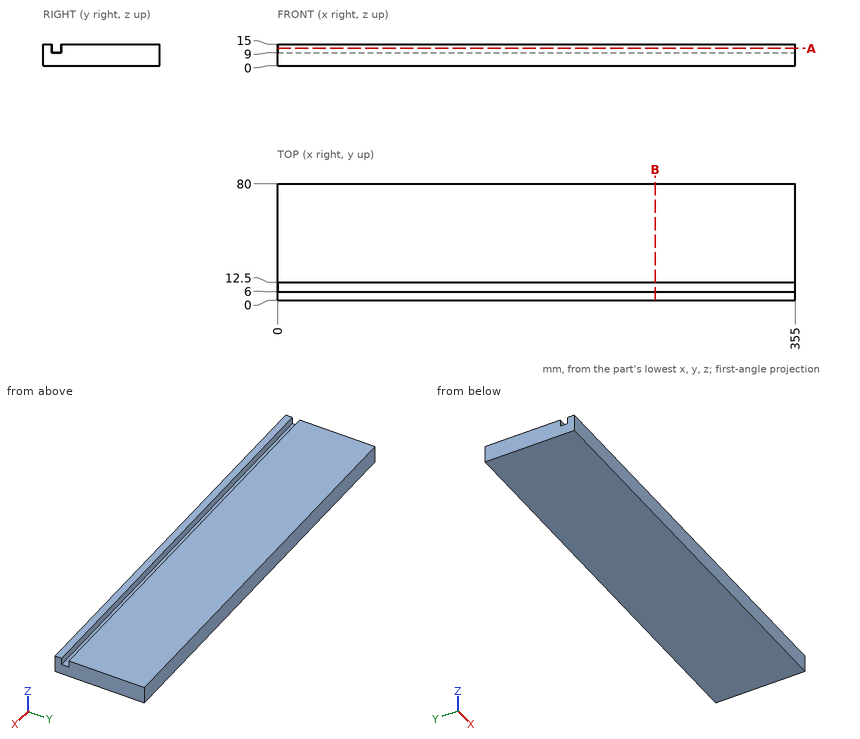
The figure shows three views and two pictorial views of one solid part (mm, origin at its lowest corner). Answer the questions. Round coordinates to 2 decimals unless told otherwise and drop trailing zeros. Loops run counter-clockwise (first coordinate to the right, second up) from the corner with the lowest first, then second, coordinate; pieces in that order, holes last. Notation, with made-up numbers: (15.25, 84.5) -> (53.25, 84.5) arc R19 cw to (53.25, 102.5) -> close; hole circle Ø10 at (-20, 7.5). An arc over 180 degrees is marked (long way). Use one line per item in the form item = value.
(1) Find section A-A on z = 12. Give the vertices of the cut face in (x, y), then the cut area to 3 significant figures.
Answer list:
outline = (0, 0) -> (355, 0) -> (355, 6) -> (0, 6) -> close; (0, 12.5) -> (355, 12.5) -> (355, 80) -> (0, 80) -> close
area = 26,100 mm2
(2) A flat-ended cylindrical pin translates along its axis: P1, Ø3, axis at x = 234.5, y = 9, coming from the +Z side. Find the tip coordinate at first contact, or state that the pin passes through.
Answer list:
P1 = 9
(3) Find section B-B on x = 259. Give the vertices of the cut face in (y, z).
Answer list:
outline = (0, 0) -> (80, 0) -> (80, 15) -> (12.5, 15) -> (12.5, 9) -> (6, 9) -> (6, 15) -> (0, 15) -> close
(4) Straight lines are drawn through the part: line 1 (Y direction, x = 127.5, z = 11); line 2 (Z direction, x = 302, y = 8). For each, find the intervals that lie inside material, in ascending order.
Answer list:
line_1 = 0 to 6, 12.5 to 80
line_2 = 0 to 9
